Can you work these out from the model? Positions are in its coordinate system, mm. Round coordinates to 2 decimals unless told otherwise and drop trailing zeros. Loops run counter-clockwise (first coordinate to the right, second up) from the corner with the lowest first, then second, coordinate; pieces in that order, holes last. Notation, with made-up numbers: M 36,3 L 60,3 A16 cw 60,23 Z; hole C -23,-24 d8. An arc over 180 degrees is marked long. Return JSON: item names as keys, results as strings.
```python
from build123d import *

# Parameters (mm, degrees)
SKETCH1_W           = 44.45
SKETCH1_H           = 39.37
BOSS_EXTRUDE1_DEPTH = 19.05
SKETCH2_R           = 11.049
CUT_EXTRUDE1_DEPTH  = 19.05
FILLET1_R           = 13.97


with BuildPart() as part:
    # Sketch1 → Boss-Extrude1 (new body)
    with BuildSketch(Plane(origin=(0, 0, 0), x_dir=(0, 0, -1), z_dir=(1, 0, 0))):
        Rectangle(SKETCH1_W, SKETCH1_H)
    extrude(amount=BOSS_EXTRUDE1_DEPTH)

    # Sketch2 → Cut-Extrude1 (cut)
    with BuildSketch(Plane(origin=(19.05, 0, 0), x_dir=(0, 0, -1), z_dir=(1, 0, 0))):
        Circle(SKETCH2_R)
    extrude(amount=-CUT_EXTRUDE1_DEPTH, mode=Mode.SUBTRACT)

    # Fillet1
    fillet1_edges = [part.edges().sort_by_distance(p)[0] for p in [
        (9.525, 19.685, 22.225),
        (9.525, 19.685, -22.225),
    ]]
    fillet(fillet1_edges, radius=FILLET1_R)


solid = part.part
```
Q1. Suppose I cut it at D-D, the plane z = 15. Please give me the cut outline in (x, y) (3 decimals), plus the area to 3 significant figures.
Results:
{"outline": "M 0,-19.685 L 19.05,-19.685 L 19.05,17.949 L 0,17.949 Z", "area": "717 mm2"}
Q2. Thinking about a two-plate mould opening in Z: for faces 1 (the flat face through (19.05, 4.7, 10.2)), 2 (the cylindrical face through (9.658, 15.484, 18.241)), 3 (the cylindrical face through (9.658, 10.955, 1.438)), which applies, pulls with the +Z half, pulls with the -Z half, needs draft (parallel to the pull), parting line crosses it, or undercut?
Results:
{"face 1": "needs draft", "face 2": "pulls with the +Z half", "face 3": "undercut"}
Q3. If I drill on line 1 along Y through (x, z) = (5.75, 0) (3 decimals); line 2 along Z through (x, y) = (13.75, 0.5) (3 decimals); line 3 along Y through (x, z) = (4.5, 5.5) (3 decimals), over which ranges is the centre line in solid material (lowest first)?
Results:
{"line 1": "y = -19.685 to -11.049, 11.049 to 19.685", "line 2": "z = -22.225 to -11.038, 11.038 to 22.225", "line 3": "y = -19.685 to -9.583, 9.583 to 19.685"}
Q4. I'm going to push flat-ended pins straight in: pin 1 Ø6 at (y, z) = (14, -2) entering from -X; pin 2 Ø5 at (x, y) = (7, 9) entering from +Z. Where does each tip first touch, or does it pass through?
Results:
{"pin 1": "stops at x = 0", "pin 2": "stops at z = 22.2"}
Q5. Suppose I cut it at B-B, the plane y = 0. Please give me the cut outline in (x, z) (3 decimals), plus the area to 3 significant figures.
Results:
{"outline": "M 0,-22.225 L 19.05,-22.225 L 19.05,-11.049 L 0,-11.049 Z; M 0,11.049 L 19.05,11.049 L 19.05,22.225 L 0,22.225 Z", "area": "426 mm2"}
Q6. Suppose I cut it at A-A, the plane z = 0. Please give me the cut outline in (x, y) (3 decimals).
Results:
{"outline": "M 0,-19.685 L 19.05,-19.685 L 19.05,-11.049 L 0,-11.049 Z; M 0,11.049 L 19.05,11.049 L 19.05,19.685 L 0,19.685 Z"}
Q7. Suppose I cut it at C-C, the plane x = 7.5. Please give me the cut outline in (y, z) (3 decimals), plus the area to 3 significant figures.
Results:
{"outline": "M -19.685,-22.225 L 5.715,-22.225 A13.97 ccw 19.685,-8.255 L 19.685,8.255 A13.97 ccw 5.715,22.225 L -19.685,22.225 Z; hole C 0,0 d22.098", "area": "1,280 mm2"}
